Autodesk Inventor part; units mm, degrees
ref_plane "YZ Plane" through (0, 0, 0) normal (1, 0, 0) x (0, 1, 0)
ref_plane "XZ Plane" through (0, 0, 0) normal (0, 1, 0) x (-1, 0, 0)
ref_plane "XY Plane" through (0, 0, 0) normal (0, 0, 1) x (1, 0, 0)
sketch "スケッチ1" plane through (0, 0, 0) normal (0, 0, 1) x (1, 0, 0)
  line L0 (0, 0) -> (0, 140)
  line L1 (0, 140) -> (0, 0)
  line L2 (0, 0) -> (48, 0)
  line L3 (48, 0) -> (48, 140)
  line L4 (48, 140) -> (0, 140)
  dimension "d0" = 140
  dimension "d1" = 48
extrude "押し出し1" add sketch "スケッチ1" along normal blind 25
fillet "フィレット1" radius 10 4 edges at (48, 70, 25) (48, 70, 0) (0, 70, 25) (0, 70, 0)
properties part number "バッテリー"
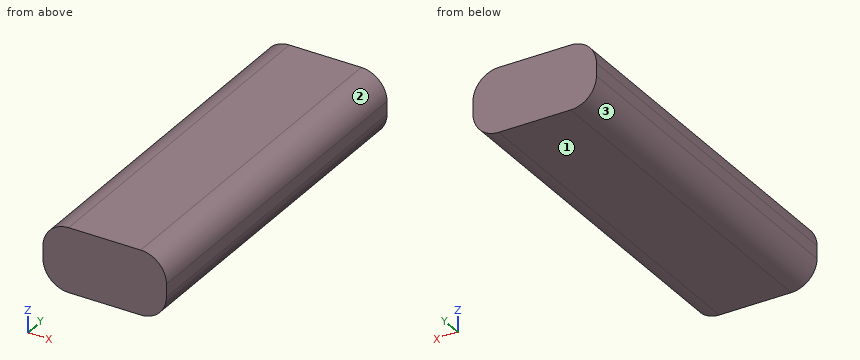
Source: CAD feature listing. Evaluate the final solid. Frame: model axes, mm. Face numbers are marked on the shaded views. Give positions to 0.01 mm unless a question says otherwise; leave off trailing zeros. Loops run counter-clockwise (first coordinate to the right, second up) from the corner with the lowest first, then second, coordinate; pieces in that order, holes last. Notation, with made-up numbers: (63, 27) - (88, 27) arc R28 cw to (88, 52) - close; hole circle Ø7 at (80, -40). An arc over 180 degrees is marked (long way). Use CSV: the item, a comma, the result in double quotes.
1) Pin query (flat end, axial travel): P1, Ø1.5, axis at y = 52, z = 4.5, coming from the +X side; P2, Ø2, axis at y = 22.5, z = 19, coming from the -X side; P3, Ø3, axis at y = 120, z = 6.5, coming from the +X side; P4, Ø3, axis at x = 33.5, z = 10.5, coming from the -Y side. Return the tip coordinate at first contact, or that it passes through.
Worked out:
P1,"stops at x = 46.8"
P2,"stops at x = 0.46"
P3,"stops at x = 47.8"
P4,"stops at y = 0"
2) Cut plane C-C (x = 42). Output: boundary loops of the cut face in (y, z), and give its area (3 significant figures).
Worked out:
outline,"(0, 0.83) - (140, 0.83) - (140, 24.17) - (0, 24.17) - close"
area,"3,270 mm^2"
3) Cut plane A-A (y = 56.5). Output: boundary loops of the cut face in (x, z).
Worked out:
outline,"(0, 10) arc R10 ccw to (10, 0) - (38, 0) arc R10 ccw to (48, 10) - (48, 15) arc R10 ccw to (38, 25) - (10, 25) arc R10 ccw to (0, 15) - close"
4) Cut plane B-B (z = 18.25). Output: boundary loops of the cut face in (x, y), and give its area (3 significant figures).
Worked out:
outline,"(0.54, 0) - (47.46, 0) - (47.46, 140) - (0.54, 140) - close"
area,"6,570 mm^2"
5) Line query: line 1 (X direction, y = 105.5, z = 19.75); line 2 (X direction, y = 27, z = 16.25); line 3 (Z direction, x = 42, y = 89.5). Output: solid intervals per line, ascending.
Worked out:
line 1,"x = 1.2 to 46.8"
line 2,"x = 0.08 to 47.92"
line 3,"z = 0.83 to 24.17"
6) Mould query, pull axis X, two halves, no side actions, for the marked faces 1, 2 and 3. Classes: +X half, -X half, draft (parallel to the pull), parting line (faces both ways), or undercut.
Worked out:
face 1,"draft"
face 2,"+X half"
face 3,"-X half"
